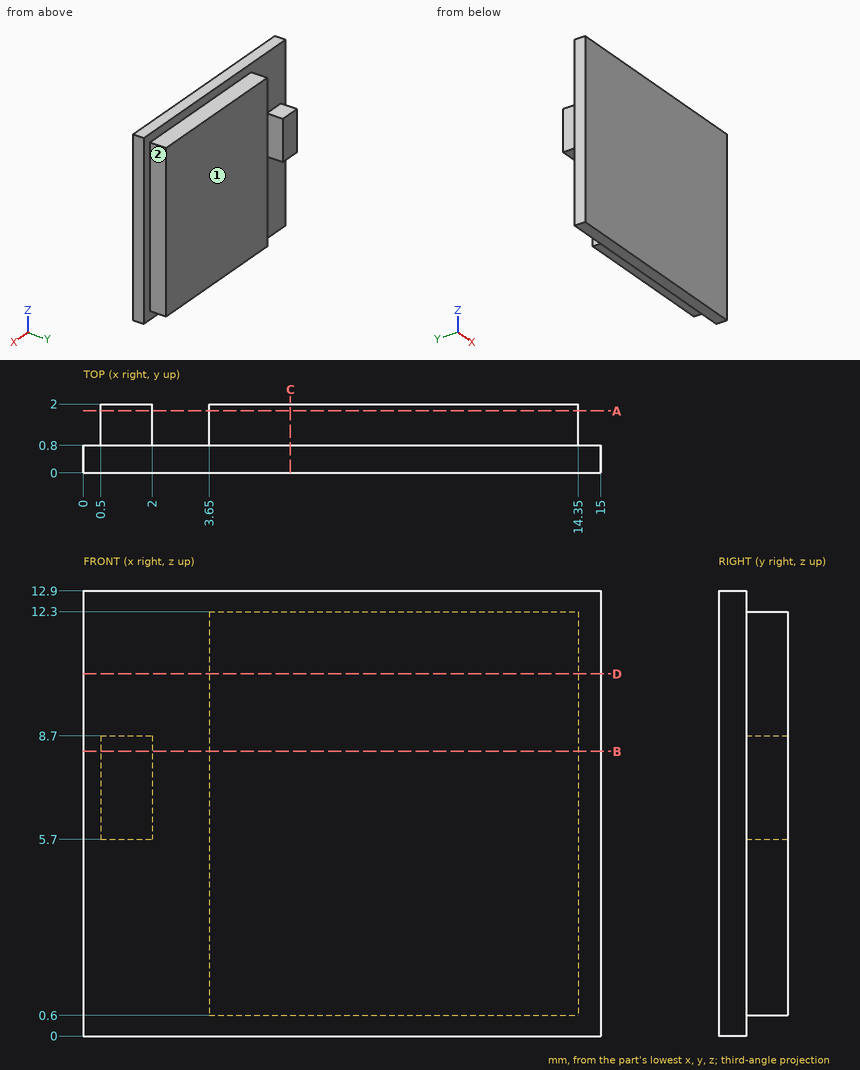
The drawing under review shows one solid part. Ordinate dimensions are in mm from its lowest x, y, z. A direction names the side the tool comes from. Round coordinates to 2 decimals unless told otherwise and drop trailing zeros. Loops run counter-clockwise (first coordinate to the right, second up) from the corner with the lowest first, then second, coordinate; pieces in that order, holes last. Notation, with made-up numbers: (18, 15) - (22, 15) arc R15 ccw to (22, 30) - close; hole circle Ø10 at (-10.75, -29). An arc over 180 degrees is marked (long way). Put each result on its own line as item: value. Start each with the question number.
1. Consider section A-A on y = 1.8. State the section outline as (x, z) points.
2. For probe 1 along Y at (x, z) = (11.5, 12.5); probe 2 along X at (y, z) = (1.85, 2.5); probe 3 along Z at (x, y) = (10.75, 1.05), list the stretches that pass through material, from the lowest coordinate up. Write a range as [from, to].
3. Insertion check: P1, Ø1, axis at x = 7.5, y = 0.5, coming from the -Z side; P2, Ø1, axis at y = 1.5, z = 7, coming from the -X side; P3, Ø0.6, axis at y = 1.5, z = 7, coming from the +X side. Each pin has a flat end and moves straight along its axis. Give the tip position at first contact, or say it passes through.
4. For the marked faces 1 and 2, list the 3-axis set-ups (+Z, -Z, +X, -X, +Y, -Y) from which the entire face can be reached by the end or side of a thin tool; tool diameter is ignored.
5. Consider section D-D on z = 10.5. State the section outline as (x, y) points, plus the area to 3 significant figures.
6. Consider section B-B on z = 8.25. State the section outline as (x, y) points, plus the area to 3 significant figures.
7. Consider section C-C on x = 6. State the section outline as (y, z) points.
Result sheet:
1. outline: (0.5, 5.7) - (2, 5.7) - (2, 8.7) - (0.5, 8.7) - close; (3.65, 0.6) - (14.35, 0.6) - (14.35, 12.3) - (3.65, 12.3) - close
2. probe 1: [0, 0.8]
2. probe 2: [3.65, 14.35]
2. probe 3: [0.6, 12.3]
3. P1: z = 0
3. P2: x = 0.5
3. P3: x = 14.35
4. face 1: +Z, -Z, +X, -X, +Y
4. face 2: +Z, -Z, +X, +Y
5. outline: (0, 0) - (15, 0) - (15, 0.8) - (14.35, 0.8) - (14.35, 2) - (3.65, 2) - (3.65, 0.8) - (0, 0.8) - close
5. area: 24.8 mm^2
6. outline: (0, 0) - (15, 0) - (15, 0.8) - (14.35, 0.8) - (14.35, 2) - (3.65, 2) - (3.65, 0.8) - (2, 0.8) - (2, 2) - (0.5, 2) - (0.5, 0.8) - (0, 0.8) - close
6. area: 26.6 mm^2
7. outline: (0, 0) - (0.8, 0) - (0.8, 0.6) - (2, 0.6) - (2, 12.3) - (0.8, 12.3) - (0.8, 12.9) - (0, 12.9) - close
